Design review of the part built by this model. Coordinates are the model's own, in mm. Coordinates: 2 decimals unless noted, no trailing zeros. Loops run counter-clockwise (first coordinate to the right, second up) from the corner with the lowest first, then second, coordinate; pieces in that order, holes last. Notation, with made-up numbers: (82, 49) -> (127, 49) arc R23 ccw to (127, 79) -> close; hole circle Ø5 at (-7.5, 71). An arc over 180 degrees is marked (long way). Use a Markdown table: item, result. Add a question column.
Q1. For probe 1 along Y at (x, z) = (-143, 6); probe 2 along X at (y, z) = (8.5, 10.5); probe 3 along X at (y, z) = (25.5, 12), list the stretches that pass through material, from the lowest coordinate up.
Q2. Take a section at A-A on x = -227. Write out the cut boundary in (y, z) (3 decimals).
Q3. Take a section at B-B on y = 49.5. Write out the cut boundary in (x, z) (3 decimals), plus the area to 3 significant figures.
Q4. Clearance check with flat-ended pins moving along their axes: pin 1 Ø1.5 at (x, z) = (-74.5, 5) entering from +Y; pin 2 Ø4 at (x, z) = (-241.5, 11.5) entering from -Y; pin 3 Ø1.5 at (x, z) = (201.5, 7.5) entering from +Y; pin 4 Ø6 at (y, z) = (16.5, 9) entering from +X. State where each tip first meets the part, or that it passes through.
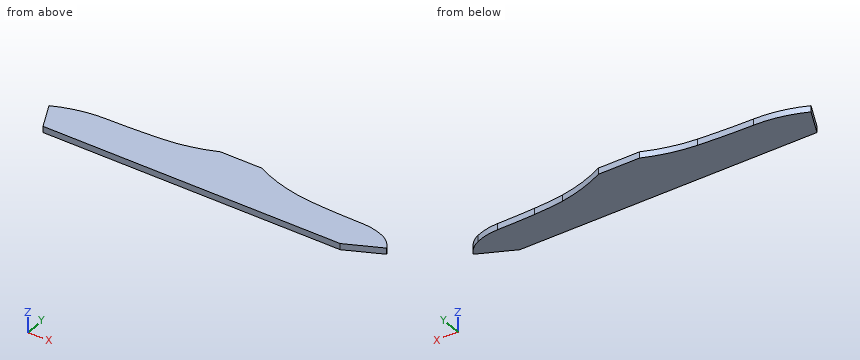
from build123d import *

# Parameters (mm, degrees)
F1_DEPTH = 15.875


with BuildPart() as f1:
    # F0 (on Top) → F1 (new body)
    with BuildSketch(Plane.XY):
        with BuildLine():
            Line((-405.7229646722, 68.1833980268), (-374.65, 0))
            Line((-374.65, 0), (374.65, 0))
            Line((374.65, 0), (464.2890758153, 40.8508803707))
            ThreePointArc((464.2890758153, 40.8508803707), (449.8955253775, 60.2323726334), (429.7637939453, 73.5564082861))
            ThreePointArc((429.7637939453, 73.5564082861), (402.1894850495, 82.3465161995), (373.4039068222, 85.3463485836))
            ThreePointArc((373.4039068222, 85.3463485837), (326.0872814579, 85.8945342918), (278.7914574146, 87.4007120728))
            add(Edge.make_bspline(
                [(202.7294188738, 94.2631438375), (213.246380745, 92.4749947437), (228.4808446175, 90.7466252174), (253.242470606, 88.7234669698), (271.076796222, 87.7246110844), (278.7914574146, 87.4007120728)],
                knots=[0, 0, 0, 0, 0.3410495495, 0.6671789133, 1, 1, 1, 1], degree=3))
            ThreePointArc((202.7294188738, 94.2631438375), (143.4379350037, 108.7622570813), (86.986720562, 131.9778710604))
            Line((86.986720562, 131.9778710604), (-16.7578142136, 131.9778710604))
            ThreePointArc((-16.7578142136, 131.9778710604), (-78.6416708287, 111.865947388), (-142.9421407222, 101.8884349303))
            ThreePointArc((-142.9421407222, 101.8884349303), (-211.4284268901, 97.9178060181), (-280.0062894821, 96.1250290275))
            ThreePointArc((-280.0062894821, 96.1250290275), (-344.3260692988, 88.7296227106), (-405.7229646722, 68.1833980268))
        make_face()
    extrude(amount=F1_DEPTH)


solid = f1.part
Answer list:
| question | item | result |
|---|---|---|
| 1 | probe 1 | 0 to 101.88 |
| 1 | probe 2 | -378.52 to 393.3 |
| 1 | probe 3 | -386.27 to 430.6 |
| 2 | outline | (0, 0) -> (97.319, 0) -> (97.319, 15.875) -> (0, 15.875) -> close |
| 3 | outline | (-397.208, 0) -> (459.137, 0) -> (459.137, 15.875) -> (-397.208, 15.875) -> close |
| 3 | area | 13,600 mm² |
| 4 | pin 1 | y = 113.06 |
| 4 | pin 2 | y = 0 |
| 4 | pin 3 | y = 94.6 |
| 4 | pin 4 | x = 417.44 |
